```python
from build123d import *

# Parameters (mm, degrees)
F0_W      = 60
F0_H      = 30
F1_DEPTH  = 60
F2_R      = 3.4
F3_DEPTH  = 60.001
F4_R      = 1.8
F5_DEPTH  = 30.001
F6_R      = 3
F7_DEPTH  = 7
F8_R      = 3
F9_DEPTH  = 7
F10_R     = 3
F11_DEPTH = 7
F12_R     = 3
F13_DEPTH = 7


with BuildPart() as f1:
    # F0 (on Top) → F1 (new body)
    with BuildSketch(Plane.XY):
        Rectangle(F0_W, F0_H)
    extrude(amount=F1_DEPTH)

    # F2 (on face) → F3 (cut, through all)
    with BuildSketch(Plane.XY.offset(60)):
        with Locations((0, 15)):
            Circle(F2_R)
    extrude(amount=-F3_DEPTH, mode=Mode.SUBTRACT)

    # F4 (on face) → F5 (cut, through all)
    with BuildSketch(Plane.XZ.offset(15)):
        with Locations((-23, 53)):
            Circle(F4_R)
        with Locations((23, 53)):
            Circle(F4_R)
        with Locations((23, 7)):
            Circle(F4_R)
        with Locations((-23, 7)):
            Circle(F4_R)
    extrude(amount=-F5_DEPTH, mode=Mode.SUBTRACT)

    # F6 (on face) → F7 (cut)
    with BuildSketch(Plane.XZ.offset(15)):
        with Locations((-23, 53)):
            Circle(F6_R)
    extrude(amount=-F7_DEPTH, mode=Mode.SUBTRACT)

    # F8 (on face) → F9 (cut)
    with BuildSketch(Plane.XZ.offset(15)):
        with Locations((23, 53)):
            Circle(F8_R)
    extrude(amount=-F9_DEPTH, mode=Mode.SUBTRACT)

    # F10 (on face) → F11 (cut)
    with BuildSketch(Plane.XZ.offset(15)):
        with Locations((-23, 7)):
            Circle(F10_R)
    extrude(amount=-F11_DEPTH, mode=Mode.SUBTRACT)

    # F12 (on face) → F13 (cut)
    with BuildSketch(Plane.XZ.offset(15)):
        with Locations((23, 7)):
            Circle(F12_R)
    extrude(amount=-F13_DEPTH, mode=Mode.SUBTRACT)


solid = f1.part
```
Design review of the part built by this model. Coordinates are the model's own, in mm. A direction names the side the tool comes from. Give positions to 0.01 mm unless a question says otherwise; leave off trailing zeros. Loops run counter-clockwise (first coordinate to the right, second up) from the corner with the lowest first, then second, coordinate; pieces in that order, holes last. Notation, with made-up numbers: (9, 82) -> (64, 82) arc R24 cw to (64, 107) -> close; hole circle Ø5 at (-23, -33.75). An arc over 180 degrees is marked (long way). One line per item, written item: value.
Q1. We need section A-A on x = -23. Give the boundary of the cut face in (y, z), and give its area (3 significant figures).
Numbers:
outline: (-15, 0) -> (15, 0) -> (15, 5.2) -> (-8, 5.2) -> (-8, 4) -> (-15, 4) -> close; (-15, 10) -> (-8, 10) -> (-8, 8.8) -> (15, 8.8) -> (15, 51.2) -> (-8, 51.2) -> (-8, 50) -> (-15, 50) -> close; (-15, 56) -> (-8, 56) -> (-8, 54.8) -> (15, 54.8) -> (15, 60) -> (-15, 60) -> close
area: 1,550 mm^2
Q2. For L1, parallel to Z at x = -23, y = -11; L2, parallel to X at y = -10.25, z = 9; L3, parallel to X at y = -4.75, z = 8, list the stretches that pass through material, from the lowest coordinate up.
Numbers:
L1: z = 0 to 4, 10 to 50, 56 to 60
L2: x = -30 to -25.24, -20.76 to 20.76, 25.24 to 30
L3: x = -30 to -24.5, -21.5 to 21.5, 24.5 to 30
Q3. Machinability: for faces 1 (the flat face through (25, -8, 53)), 2 (the flat face through (0, 0, 0)), which of the approach directions +Z, -Z, +X, -X, +Y, -Y give a long, thin tool a straight path to every point of the face, cutting with its end or side? Answer none if there is none.
Numbers:
face 1: -Y
face 2: -Z, +X, -X, +Y, -Y
Q4. Draft analysis for pull direction X (two halves, no side actions). For faces 3 (the flat face through (-30, 0, 30)), 4 (the flat face through (25, -8, 7)), 5 (the flat face through (0, 0, 60)), state which applies: pulls with the +X half, pulls with the -X half, needs draft (parallel to the pull), parting line crosses it, or undercut.
Numbers:
face 3: pulls with the -X half
face 4: undercut
face 5: needs draft
Q5. We need section C-C on x = 0. Give the boundary of the cut face in (y, z), and give its area (3 significant figures).
Numbers:
outline: (-15, 0) -> (11.6, 0) -> (11.6, 60) -> (-15, 60) -> close
area: 1,600 mm^2
Q6. For pin 1 Ø12 at (x, y) = (-3, 3.5) entering from -Z; pin 2 Ø1.5 at (x, z) = (0, 33.5) entering from +Y; pin 3 Ø1.8 at (x, z) = (24, 7.5) entering from -Y, all flat-tipped, find the tip position at first contact; note any pin that passes through.
Numbers:
pin 1: stops at z = 0
pin 2: stops at y = 11.68
pin 3: stops at y = -8
Q7. We need section B-B on z = 53. Give the boundary of the cut face in (x, y).
Numbers:
outline: (-30, -15) -> (-26, -15) -> (-26, -8) -> (-24.8, -8) -> (-24.8, 15) -> (-30, 15) -> close; (-21.2, -8) -> (-20, -8) -> (-20, -15) -> (20, -15) -> (20, -8) -> (21.2, -8) -> (21.2, 15) -> (3.4, 15) arc R3.4 cw to (-3.4, 15) -> (-21.2, 15) -> close; (24.8, -8) -> (26, -8) -> (26, -15) -> (30, -15) -> (30, 15) -> (24.8, 15) -> close
